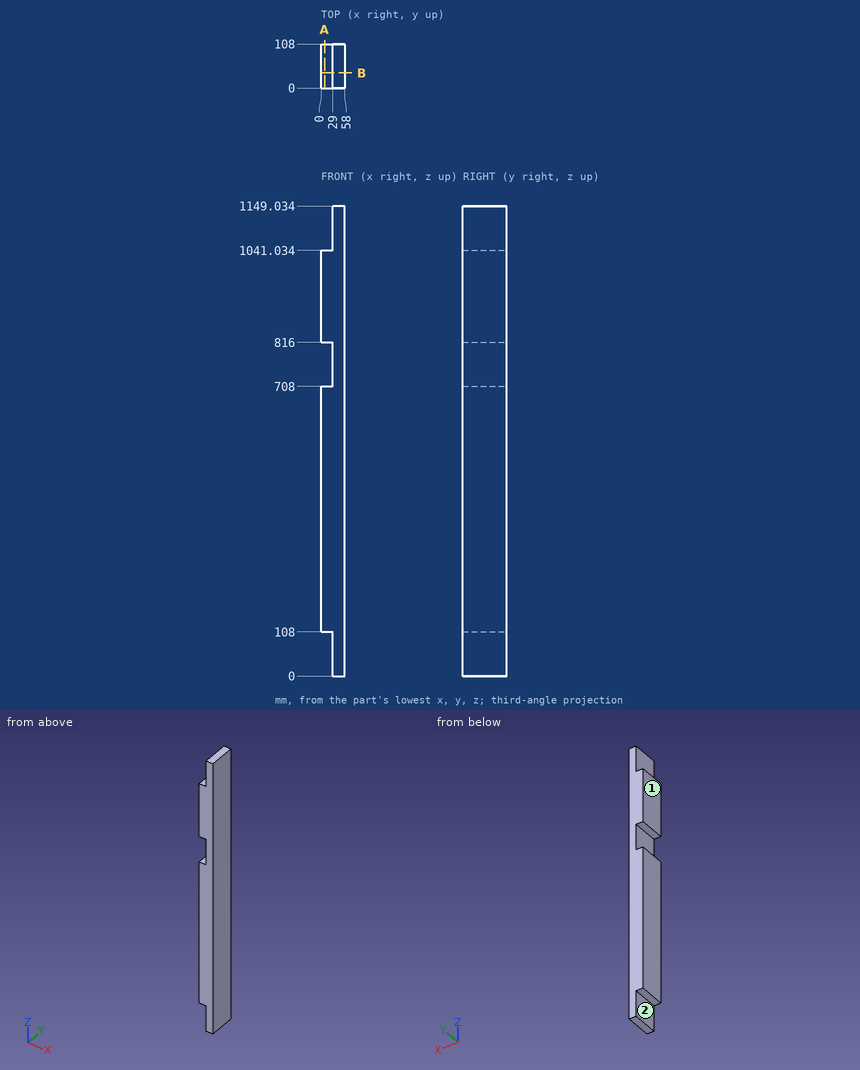
Input: dimensioned drawing with shaded views. Units: mm. Origin: part minimum x, y, z. A direction names the side the tool comes from. Coordinates: 2 decimals unless noted, no trailing zeros. Order: outer loops, then holes, each group sorted by start corner. A loop starts at its lowest first (then second) coordinate and runs counter-clockwise, first axis right, second up. Notation, with made-up numbers: M 77,43.5 L 109,43.5 A8 ccw 109,56.5 Z; hole C 2.5,12.5 d11. An arc over 180 degrees is marked long. Write each question's results on one line, items separated by ' | '. Start each with the question number.
Item 1: First-contact query: pin 1 Ø2 at (x, y) = (10, 54) entering from +Z; pin 2 Ø14.5 at (x, y) = (9, 36) entering from -Z; pin 3 Ø10 at (x, z) = (10.5, 1016) entering from -Y. Flat tips, straight axial feed; report the tip coordinate or a pass-through.
Item 2: Cut plane B-B (y = 37.5). Return loops of the section in (x, z), and give its area (3 significant figures).
Item 3: Cut plane A-A (x = 9). Return loops of the section in (y, z).
Item 4: Line query: probe 1 along Z at (x, y) = (22, 82.5); probe 2 along X at (y, z) = (38, 806). Output: solid intervals per line, ascending.
Item 5: Set-up query: the marked faces 1 and 2. Return all of +Z, -Z, +X, -X, +Y, -Y with unobstructed straight access to the full face (end or side cutting, diameter ignored); none if empty.
Checked values:
1) pin 1: stops at z = 1041.03 | pin 2: stops at z = 108 | pin 3: stops at y = 0
2) outline: M 0,108 L 29,108 L 29,0 L 58,0 L 58,1149.03 L 29,1149.03 L 29,1041.03 L 0,1041.03 L 0,816 L 29,816 L 29,708 L 0,708 Z | area: 57,200 mm2
3) outline: M 0,108 L 108,108 L 108,708 L 0,708 Z; M 0,816 L 108,816 L 108,1041.03 L 0,1041.03 Z
4) probe 1: z = 108 to 708, 816 to 1041.03 | probe 2: x = 29 to 58
5) face 1: +Z, -Z, -X, +Y, -Y | face 2: -Z, -X, +Y, -Y
